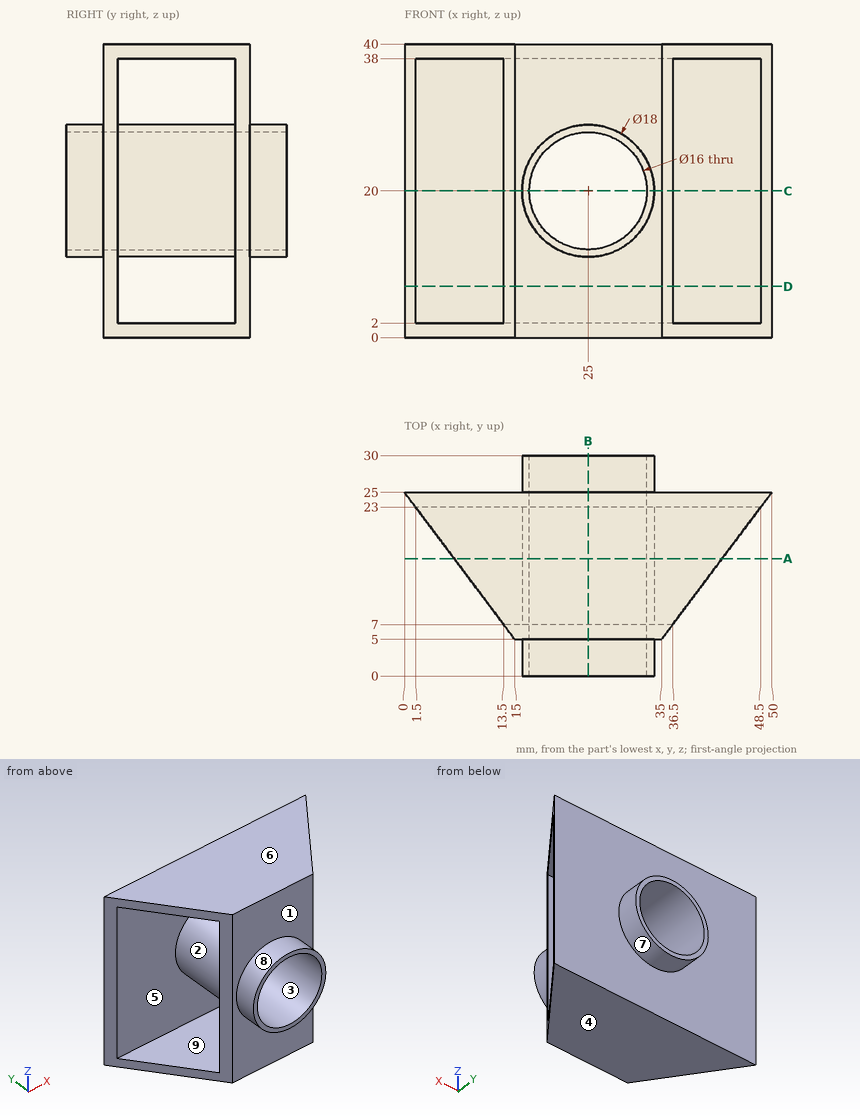
Verification items for this drawing (mm, ordinates from the low corner). A direction names the side the tool comes from. Coordinates: 2 decimals unless noted, no trailing zeros. Loops run counter-clockwise (first coordinate to the right, second up) from the corner with the lowest first, then second, coordinate; pieces in that order, holes last. Notation, with made-up numbers: (85.5, 41) - (116.5, 41) arc R12 ccw to (116.5, 60) - close; hole circle Ø5 at (28.25, 13.5). An arc over 180 degrees is marked (long way). One line per item, written item: value. Start each with the question number.
(1) Cross-section at C-C on z = 20. Enter the section's corners in (x, y), plus the area to 3 significant figures.
(2) Tool access check on the marked faces 5, 6, 7, 8 and 9. Record the directions out of +Z, -Z, +X, -X, +Y, -Y that give a thin tool (end or side, any length) a straight path to the whole face; none if there is none.
(3) Cross-section at A-A on y = 16. Enter the section's corners in (x, z), plus the area to 3 significant figures.
(4) Material ranges on line 1 (Z direction, x = 36, y = 22.25); line 2 (X direction, y = 11.5, z = 20); line 3 (Y direction, x = 19, z = 7.5), recorded low to high. Write a range as [from, to].
(5) Cross-section at D-D on z = 7. Enter the section's corners in (x, y), plus the area to 3 significant figures.
(6) Depth check by flat-ended pin: P1, Ø8, axis at y = 20.5, z = 22.5, coming from the +X side (3 decimals); P2, Ø12, axis at y = 18.5, z = 4.5, coming from the -X side (3 decimals); P3, Ø14.5, axis at x = 25, z = 20, coming from the +Y side; P4, Ø2, axis at x = 19.5, z = 5.5, coming from the +Y side. Enter the tip coordinate at first touch or a pass-through.
(7) Cross-section at B-B on x = 25. Enter the section's corners in (y, z).
(8) Mould release check, pull along Z, two halves, no side actions. Record for the marked faces 1, 2, 3 and 4: released by +Z, released by -Z, zero draft, split by the parting line, or undercut.
Results below:
1. outline: (0, 25) - (1.5, 23) - (16, 23) - (16, 7) - (13.5, 7) - (15, 5) - (16, 5) - (16, 0) - (17, 0) - (17, 30) - (16, 30) - (16, 25) - close; (33, 0) - (34, 0) - (34, 5) - (35, 5) - (36.5, 7) - (34, 7) - (34, 23) - (48.5, 23) - (50, 25) - (34, 25) - (34, 30) - (33, 30) - close
1. area: 128 mm2
2. face 5: none
2. face 6: +Z, +X, -X, +Y, -Y
2. face 7: +Y
2. face 8: -Y
2. face 9: +X, -X
3. outline: (6.75, 0) - (43.25, 0) - (43.25, 2) - (6.75, 2) - close; (6.75, 38) - (43.25, 38) - (43.25, 40) - (6.75, 40) - close; circle Ø18 at (25, 20); hole circle Ø16 at (25, 20)
3. area: 199 mm2
4. line 1: z = [0, 2], [38, 40]
4. line 2: x = [16, 17], [33, 34]
4. line 3: y = [5, 7], [23, 25]
5. outline: (0, 25) - (1.5, 23) - (48.5, 23) - (50, 25) - close; (13.5, 7) - (15, 5) - (35, 5) - (36.5, 7) - close
5. area: 140 mm2
6. P1: stops at x = 49.625
6. P2: stops at x = 0.375
6. P3: passes through
6. P4: stops at y = 25
7. outline: (0, 11) - (5, 11) - (5, 0) - (25, 0) - (25, 11) - (30, 11) - (30, 12) - (0, 12) - close; (0, 28) - (30, 28) - (30, 29) - (25, 29) - (25, 40) - (5, 40) - (5, 29) - (0, 29) - close; hole (7, 2) - (23, 2) - (23, 11) - (7, 11) - close; hole (7, 29) - (23, 29) - (23, 38) - (7, 38) - close
8. face 1: zero draft
8. face 2: undercut
8. face 3: undercut
8. face 4: released by -Z
